Source: three-view drawing plus pictorial views. Frame: mm from the lowest corner of the part. Give positions to 0.01 mm unless a question says otherwise; leave off trailing zeros. Write each loop counter-clockwise with the first axis right and the second up, starting at its lowest first coordinate (ties: lowest second). Pieces come first, ordered by that corner, then holes.
Q1. Line query: L1, parallel to Y at x = 3.2, z = 53.5 (1 decimal); L2, parallel to Y at x = 0.6, z = 4 (1 decimal); L3, parallel to Z at x = 4.7, y = 49.5 (1 decimal). Output: solid intervals per line, ascending.
Q2. Pin query (flat end, axial travel): pin 1 (13 mm diameter, centred on y = 10, z = 10, fed in from +X); pin 2 (1 mm diameter, centred on x = 1.5, y = 33, fed in from -Z); pin 3 (2 mm diameter, centred on x = 2, z = 36.5, fed in from -Y); pin 4 (3 mm diameter, centred on x = 3.5, y = 35.5, fed in from +Z). Return the tip coordinate at first contact, or that it passes through.
Q3. Cut plane A-A on z = 10. Return the cut outline in (x, y).
Q4. Draft query along Z for the marked faces 1, 2 and 3. Return one class per face: pulls with the +Z half, pulls with the -Z half, needs draft (parallel to the pull), parting line crosses it, or undercut.
Q5. Cut plane D-D on z = 34. Return the cut outline in (x, y) (1 decimal), plus the area to 3 significant figures.
Q6. Cut plane C-C on x = 2.7. Return the cut outline in (y, z) (1 decimal).
Q7. Cut plane B-B on y = 12.5. Return the cut outline in (x, z).
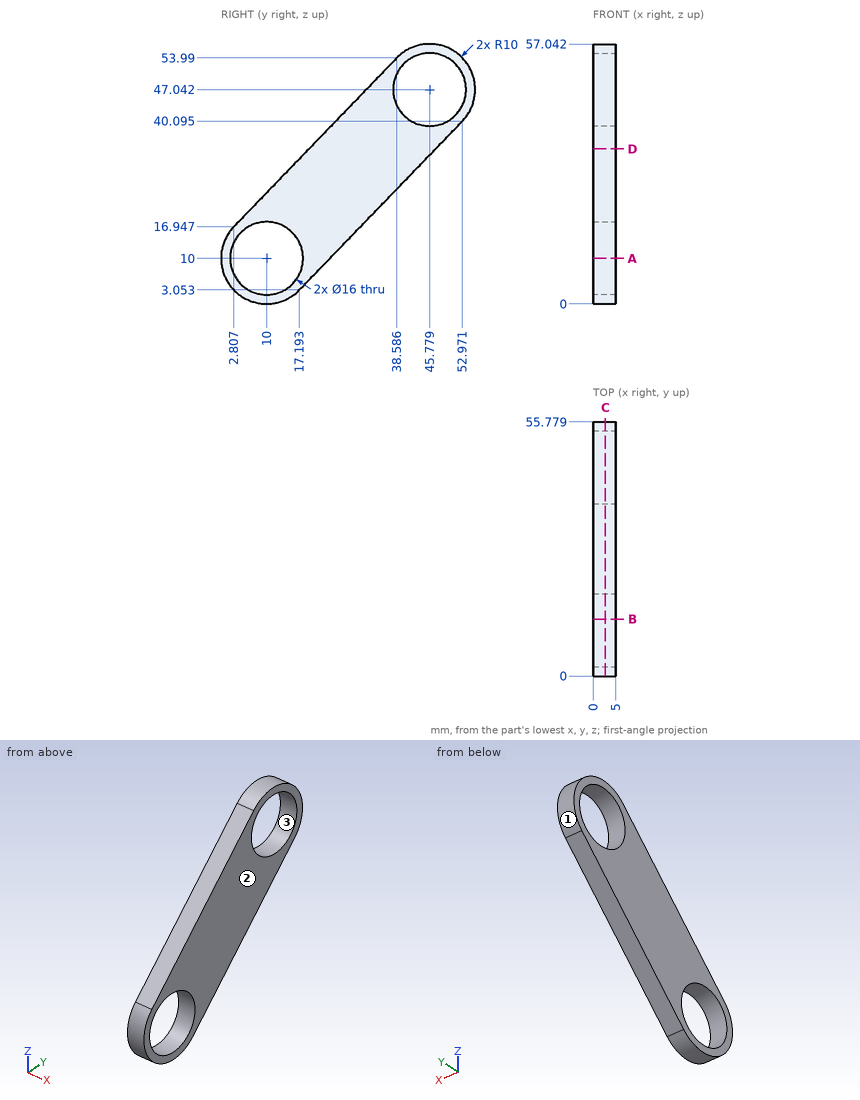
Data:
1. L1: y = 38.1 to 41.1, 50.5 to 53.4
1. L2: y = 2 to 4.7, 15.3 to 18.1
1. L3: z = 36.5 to 40, 54.1 to 56.3
2. pin 1: passes through
2. pin 2: stops at z = 18.9
2. pin 3: stops at y = 20.73
2. pin 4: stops at z = 52.35
3. outline: (0, 0) - (5, 0) - (5, 2) - (0, 2) - close; (0, 18) - (5, 18) - (5, 23.9) - (0, 23.9) - close
4. face 1: parting line crosses it
4. face 2: needs draft
4. face 3: undercut
5. outline: (0, 19.3) - (5, 19.3) - (5, 47.1) - (0, 47.1) - close
5. area: 139 mm2
6. outline: (2.8, 16.9) arc R10 ccw to (17.2, 3.1) - (53, 40.1) arc R10 ccw to (38.6, 54) - close; hole circle Ø16 at (10, 10); hole circle Ø16 at (45.8, 47)
7. outline: (0, 0.32) - (5, 0.32) - (5, 2.4) - (0, 2.4) - close; (0, 17.6) - (5, 17.6) - (5, 26.98) - (0, 26.98) - close
